from build123d import *

# Parameters (mm, degrees)
SKETCH_1_W          = 57
SKETCH_1_H          = 45
EXTRUDE_1_DEPTH     = 3
SKETCH_2_W          = 4
SKETCH_2_H          = 15
EXTRUDE_2_DEPTH     = 6
SKETCH_3_W          = 4
SKETCH_3_H          = 15
EXTRUDE_3_DEPTH     = 6
EXTRUDE_4_DEPTH     = 3
SKETCH_5_W          = 4
SKETCH_5_H          = 9
EXTRUDE_5_DEPTH     = 3
CHAMFER_1_SIZE      = 3
SKETCH_6_R          = 1.6
CUT_EXTRUDE_1_DEPTH = 4
SKETCH_7_R          = 1.6
CUT_EXTRUDE_2_DEPTH = 3
SKETCH_8_W          = 8
SKETCH_8_H          = 3
EXTRUDE_6_DEPTH     = 9
EXTRUDE_7_DEPTH     = 3
EXTRUDE_8_DEPTH     = 3
SKETCH_11_R         = 1.6
CUT_EXTRUDE_3_DEPTH = 3
SKETCH_12_W         = 5
SKETCH_12_H         = 17
CUT_EXTRUDE_4_DEPTH = 3
FILLET_1_R          = 1.5


with BuildPart() as part:
    # 草图1 → 凸台-拉伸1 (new body)
    with BuildSketch(Plane(origin=(0, 0, 0), x_dir=(1, 0, 0), z_dir=(0, 1, 0))):
        with Locations((28.5, 22.5)):
            Rectangle(SKETCH_1_W, SKETCH_1_H)
    extrude(amount=EXTRUDE_1_DEPTH)

    # 草图2 → 凸台-拉伸2 (add)
    with BuildSketch(Plane.ZY):
        with Locations((-2, -1.5)):
            Rectangle(SKETCH_2_W, SKETCH_2_H)
    extrude(amount=EXTRUDE_2_DEPTH)

    # 草图3 → 凸台-拉伸3 (add)
    with BuildSketch(Plane(origin=(57, 0, 0), x_dir=(0, 0, -1), z_dir=(1, 0, 0))):
        with Locations((2, -1.5)):
            Rectangle(SKETCH_3_W, SKETCH_3_H)
    extrude(amount=EXTRUDE_3_DEPTH)

    # 草图4 → 凸台-拉伸4 (add)
    with BuildSketch(Plane.ZY.offset(-57)):
        Polygon((-4, -9), (-19.588457268, 0), (0, 0), (0, -9), align=None)
    extrude(amount=EXTRUDE_4_DEPTH)

    # 草图5 → 凸台-拉伸5 (add)
    with BuildSketch(Plane(origin=(0, 0, 0), x_dir=(0, 0, -1), z_dir=(1, 0, 0))):
        Polygon((19.588457268, 0), (4, 0), (4, -9), align=None)
        with Locations((2, -4.5)):
            Rectangle(SKETCH_5_W, SKETCH_5_H)
    extrude(amount=EXTRUDE_5_DEPTH)

    # 倒角1
    chamfer_1_edges = [part.edges().sort_by_distance(p)[0] for p in [
        (0, 3, -2),
        (57, 3, -2),
    ]]
    chamfer(chamfer_1_edges, length=CHAMFER_1_SIZE - 0.0001)  # a hair under: the kernel refuses the full size

    # 草图6 → 切除-拉伸1 (cut)
    with BuildSketch(Plane(origin=(0, 0, -4), x_dir=(-1, 0, 0), z_dir=(0, 0, -1))):
        with Locations(Location((3, -2.323268139, 0), (0, 0, 90))):
            Circle(SKETCH_6_R)
        with Locations(Location((-60, -2.323268139, 0), (0, 0, 90))):
            Circle(SKETCH_6_R)
    extrude(amount=-CUT_EXTRUDE_1_DEPTH, mode=Mode.SUBTRACT)

    # 草图7 → 切除-拉伸2 (cut)
    with BuildSketch(Plane(origin=(0, 3, 0), x_dir=(1, 0, 0), z_dir=(0, 1, 0))):
        with Locations(Location((8, 41, 0), (0, 0, 270))):
            Circle(SKETCH_7_R)
        with Locations(Location((8, 4, 0), (0, 0, 270))):
            Circle(SKETCH_7_R)
        with Locations(Location((48, 4, 0), (0, 0, 270))):
            Circle(SKETCH_7_R)
        with Locations(Location((48, 41, 0), (0, 0, 270))):
            Circle(SKETCH_7_R)
    extrude(amount=-CUT_EXTRUDE_2_DEPTH, mode=Mode.SUBTRACT)

    # 草图8 → 凸台-拉伸6 (add)
    with BuildSketch(Plane.XZ):
        with Locations((28, -43.5)):
            Rectangle(SKETCH_8_W, SKETCH_8_H)
    extrude(amount=EXTRUDE_6_DEPTH)

    # 草图9 → 凸台-拉伸7 (add)
    with BuildSketch(Plane(origin=(32, 0, 0), x_dir=(0, 0, -1), z_dir=(1, 0, 0))):
        Polygon((45, 0), (29.146667939, 0), (42, -9), (45, -9), align=None)
    extrude(amount=EXTRUDE_7_DEPTH)

    # 草图10 → 凸台-拉伸8 (add)
    with BuildSketch(Plane.ZY.offset(-24)):
        Polygon((-45, 0), (-45, -9), (-42, -9), (-29.146667939, 0), align=None)
    extrude(amount=EXTRUDE_8_DEPTH)

    # 草图11 → 切除-拉伸3 (cut)
    with BuildSketch(Plane.XY.offset(-42)):
        with Locations((28, -4.5)):
            Circle(SKETCH_11_R)
    extrude(amount=-CUT_EXTRUDE_3_DEPTH, mode=Mode.SUBTRACT)

    # 草图12 → 切除-拉伸4 (cut)
    with BuildSketch(Plane(origin=(0, 3, 0), x_dir=(1, 0, 0), z_dir=(0, 1, 0))):
        with Locations((28, 19)):
            Rectangle(SKETCH_12_W, SKETCH_12_H)
    extrude(amount=-CUT_EXTRUDE_4_DEPTH, mode=Mode.SUBTRACT)

    # 圆角1
    fillet_1_edges = [part.edges().sort_by_distance(p)[0] for p in [
        (25.5, 1.5, -27.5),
        (30.5, 1.5, -27.5),
        (30.5, 1.5, -10.5),
        (25.5, 1.5, -10.5),
    ]]
    fillet(fillet_1_edges, radius=FILLET_1_R)


solid = part.part
For this review, take the finished solid that the model builds, in its own axes (mm). A direction names the side the tool comes from. Give positions to 0.01 mm unless a question says otherwise; leave off trailing zeros. Loops run counter-clockwise (first coordinate to the right, second up) from the corner with the lowest first, then second, coordinate; pieces in that order, holes last. Notation, with made-up numbers: M 55,42 L 61,42 A25 cw 61,73 Z; hole C 77,78 d11. An arc over 180 degrees is marked long. Put each result on its own line as item: value. Start each with the question number.
(1) Wall thickness on L1, parallel to X at y = -3, z = -38; L2, parallel to Y at x = 28, z = -43; L3, parallel to X at y = 1, z = -42: over which ranges is each line inside the solid? List them lowest first.
(2) For pin 1 (2 mm diameter, centred on y = -3, z = -37.5, fed in from -X); pin 2 (0.9 mm diameter, centred on y = 2, z = -19.5, fed in from -X); pin 3 (10 mm diameter, centred on x = 48.5, z = -18.5, fed in from -Y), all flat-tipped, find the tip position at first contact; note any pin that passes through.
(3) The part is to be moulded in two halves that separate along X. For faces 5 (the cylindrical face through (49.35, 1.52, -3.14)), 6 (the flat face through (63, -1, -2)), 7 (the flat face through (59, -9, -2)), say which applies: +X half, -X half, draft (parallel to the pull), parting line (faces both ways), or undercut.
(4) Machinability: for faces 1 (the flat face through (56, 5, -2)), 2 (the flat face through (54, -3, -7)), 3 (the flat face through (28, 2, -10.5)), 4 (the flat face through (32, -2, -38)), which of the approach directions +Z, -Z, +X, -X, +Y, -Y give a long, thin tool a straight path to every point of the face, cutting with its end or side? Answer none if there is none.
(5) Add section B-B, the plane x = 8. Write out the cut boundary in (y, z).
(6) Add section A-A, the plane y = 1.5. Write out the cut boundary in (x, z), then the cut area to 3 significant figures.
(7) Add section D-D, the plane x = -3. Write out the cut boundary in (y, z), then the cut area to 3 significant figures.
(8) Add section C-C, the plane z = -15.5. Write out the cut boundary in (x, y).
Result:
1. L1: x = 21 to 24, 32 to 35
1. L2: y = -9 to -6.1, -2.9 to 3
1. L3: x = 0 to 6.75, 9.25 to 46.75, 49.25 to 57
2. pin 1: stops at x = 21
2. pin 2: stops at x = 0
2. pin 3: stops at y = 0
3. face 5: undercut
3. face 6: +X half
3. face 7: draft
4. face 1: +Z, -Z, +Y
4. face 2: +Z, -Z, -Y
4. face 3: +Y, -Y
4. face 4: +Z, -Y
5. outline: M 0,-45 L 3,-45 L 3,-42.6 L 0,-42.6 Z; M 0,-39.4 L 3,-39.4 L 3,-5.6 L 0,-5.6 Z; M 0,-2.4 L 3,-2.4 L 3,0 L 0,0 Z
6. outline: M -6,-4 L 0,-4 L 0,-45 L 57,-45 L 57,-4 L 63,-4 L 63,0 L -6,0 Z; hole C 8,-41 d3.2; hole C 8,-4 d3.2; hole M 25.5,-26 A1.5 ccw 27,-27.5 L 29,-27.5 A1.5 ccw 30.5,-26 L 30.5,-12 A1.5 ccw 29,-10.5 L 27,-10.5 A1.5 ccw 25.5,-12 Z; hole C 48,-41 d3.2; hole C 48,-4 d3.2
6. area: 2,500 mm^2
7. outline: M -9,-4 L -3.92,-4 L -3.92,0 L -9,0 Z; M -0.72,-4 L 6,-4 L 6,0 L -0.72,0 Z
7. area: 47.2 mm^2
8. outline: M 0,-2.36 L 3,-2.36 L 3,0 L 25.5,0 L 25.5,3 L 0,3 Z; M 30.5,0 L 54,0 L 54,-2.36 L 57,-2.36 L 57,3 L 30.5,3 Z
